Build history of the part. All positions in model axes, mm. A direction names the side the tool comes from. Give positions to 0.01 mm unless a question says otherwise; leave off trailing zeros. Use a Markdown table: item, result. Add a question column.
(1) Which spindle directions (+Z, -Z, +X, -X, +Y, -Y) get a long thin tool onto all of the face, cutting with end or side? Do faces 1 (the face through (20.2, 17.72, 11.43)), 2 (the face through (-18.88, 17.75, -11.4)), 3 (the face through (21, 18.322, 0)), 4 (the face through (24.7, 9.29, -4.72)), 5 (the face through (20.4, 17.72, -11.43)). Say none if no direction does.
(2) Flat gauge pins, fed straight in: pin 1 (1 mm diameter, centred on x = -1.5, z = -6.5, fed in from -Y); pin 2 (12 mm diameter, centred on x = 14.5, y = 6.5, fed in from -Z); pin 3 (3.5 mm diameter, centred on x = 24.15, z = 7, fed in from -Y); pin 4 (4 mm diameter, centred on x = 23.5, z = 2, fed in from +Y). Where does each tip first touch, or does it go through?
(3) Wall check: line 1 (Z direction, x = -21.15, y = 6); line 2 (Z direction, x = 24.15, y = 9.25); line 3 (X direction, y = 14.75, z = -4.25). Give the ranges that are in metal, low to high.
(4) Slice it at A-A (y = 8.75). Count the separate pieces of the cut face and the enclosed holes in it, then the cut area to 3 significant figures.
from build123d import *

# Parameters (mm, degrees)
AUFSATZ_LINEAR_AUSTRAGEN1_DEPTH = 12
SKIZZE2_R                       = 2.25
SCHNITT_LINEAR_AUSTRAGEN1_DEPTH = 19.322117782
SCHNITT_LINEAR_AUSTRAGEN2_DEPTH = 19.322117782
SCHNITT_LINEAR_AUSTRAGEN3_DEPTH = 19.322117782
VERRUNDUNG1_R                   = 2
VERRUNDUNG2_R                   = 2


with BuildPart() as part:
    # Skizze1 → Aufsatz-Linear austragen1 (new body, symmetric)
    with BuildSketch(Plane.XY):
        with BuildLine():
            ThreePointArc((18.31643729, 10.575), (20.429331226, 5.474022804), (21.15, 0))
            Line((21.15, 0), (29.15, 0))
            Line((29.15, 0), (29.15, 18.322117782))
            Line((29.15, 18.322117782), (14.15, 18.322117782))
            ThreePointArc((14.15, 18.322117782), (0, 23.15), (-14.15, 18.322117782))
            Line((-14.15, 18.322117782), (-26.15, 18.322117782))
            Line((-26.15, 18.322117782), (-26.15, 0))
            Line((-26.15, 0), (-16.15, 0))
            ThreePointArc((-16.15, 0), (-6.544357391, 14.764616024), (10.846146915, 11.965934861))
            ThreePointArc((10.846146915, 11.965934861), (14.901557957, 12.990518454), (18.31643729, 10.575))
        make_face()
    extrude(amount=AUFSATZ_LINEAR_AUSTRAGEN1_DEPTH, both=True)

    # Skizze2 → Schnitt-Linear austragen1 (cut, through all)
    with BuildSketch(Plane(origin=(0, 18.322117782, 0), x_dir=(1, 0, 0), z_dir=(0, 1, 0))):
        with Locations((-21.15, 6.5)):
            Circle(SKIZZE2_R)
        with BuildLine():
            Line((-22.275, 4.551442841), (-21.15, 3.901923789))
            Line((-21.15, 3.901923789), (-20.025, 4.551442841))
            ThreePointArc((-20.025, 4.551442841), (-21.15, 4.25), (-22.275, 4.551442841))
        make_face()
    extrude(amount=-SCHNITT_LINEAR_AUSTRAGEN1_DEPTH, mode=Mode.SUBTRACT)

    # Skizze2_4 → Schnitt-Linear austragen2 (cut, through all)
    with BuildSketch(Plane(origin=(0, 18.322117782, 0), x_dir=(1, 0, 0), z_dir=(0, 1, 0))):
        with BuildLine():
            Line((23.025, 5.051442841), (24.15, 4.401923789))
            Line((24.15, 4.401923789), (25.275, 5.051442841))
            ThreePointArc((25.275, 5.051442841), (24.15, 9.25), (23.025, 5.051442841))
        make_face()
    extrude(amount=-SCHNITT_LINEAR_AUSTRAGEN2_DEPTH, mode=Mode.SUBTRACT)

    # Skizze2_5 → Schnitt-Linear austragen3 (cut, through all)
    with BuildSketch(Plane(origin=(0, 18.322117782, 0), x_dir=(1, 0, 0), z_dir=(0, 1, 0))):
        with BuildLine():
            Line((23.025, -8.948557159), (24.15, -9.598076211))
            Line((24.15, -9.598076211), (25.275, -8.948557159))
            ThreePointArc((25.275, -8.948557159), (24.15, -4.75), (23.025, -8.948557159))
        make_face()
        with BuildLine():
            Line((-22.275, -8.948557159), (-21.15, -9.598076211))
            Line((-21.15, -9.598076211), (-20.025, -8.948557159))
            ThreePointArc((-20.025, -8.948557159), (-21.15, -4.75), (-22.275, -8.948557159))
        make_face()
    extrude(amount=-SCHNITT_LINEAR_AUSTRAGEN3_DEPTH, mode=Mode.SUBTRACT)

    # Verrundung1
    verrundung1_edges = [part.edges().sort_by_distance(p)[0] for p in [
        (20.429331226, 5.474022804, 12),
        (-6.544357391, 14.764616024, -12),
        (-26.15, 9.161058891, -12),
        (29.15, 9.161058891, -12),
        (20.429331226, 5.474022804, -12),
        (14.901557957, 12.990518454, -12),
        (10.846146915, 11.965934861, 0),
        (29.15, 9.161058891, 12),
        (-26.15, 9.161058891, 12),
        (-6.544357391, 14.764616024, 12),
        (14.901557957, 12.990518454, 12),
    ]]
    fillet(verrundung1_edges, radius=VERRUNDUNG1_R)

    # Verrundung2
    verrundung2_edges = [part.edges().sort_by_distance(p)[0] for p in [
        (-26.15, 18.322117782, 0),
        (-25.564213562, 18.322117782, 11.414213562),
        (-25.564213562, 18.322117782, -11.414213562),
        (0, 23.15, -12),
        (0, 23.15, 12),
        (20.65, 18.322117782, 12),
        (-19.15, 18.322117782, 12),
        (-19.15, 18.322117782, -12),
        (20.65, 18.322117782, -12),
        (29.15, 18.322117782, 0),
        (28.564213562, 18.322117782, 11.414213562),
        (28.564213562, 18.322117782, -11.414213562),
    ]]
    fillet(verrundung2_edges, radius=VERRUNDUNG2_R)


solid = part.part
Solution:
| question | item | result |
|---|---|---|
| 1 | face 1 | +Z, +X, +Y |
| 1 | face 2 | -Z, -X, +Y |
| 1 | face 3 | +Z, -Z, +X, +Y |
| 1 | face 4 | +Y, -Y |
| 1 | face 5 | -Z, +X, +Y |
| 2 | pin 1 | y = 16.03 |
| 2 | pin 2 | z = -11.55 |
| 2 | pin 3 | through |
| 2 | pin 4 | y = 18.32 |
| 3 | line 1 | -12 to -8.75, -3.9 to 4.75, 9.6 to 12 |
| 3 | line 2 | -12 to -9.25, -4.4 to 4.75, 9.6 to 12 |
| 3 | line 3 | -26.15 to -21.75, -20.55 to -6.58, 6.58 to 29.15 |
| 4 | separate pieces | 2 |
| 4 | enclosed holes | 4 |
| 4 | area | 467 mm2 |
